Source: three-view drawing plus pictorial views. Frame: mm from the lowest corner of the part. Coordinates: 2 decimals unless noted, no trailing zeros. Write each loop counter-clockwise with the first axis right and the second up, starting at its lowest first coordinate (ties: lowest second). Pieces come first, ordered by that corner, then holes. Notation, with made-up numbers: (81.5, 68.5) -> (120.5, 68.5) arc R19 ccw to (120.5, 83.5) -> close; hole circle Ø10 at (3, -5). An arc over 180 degrees is marked (long way). One line per item, written item: value.
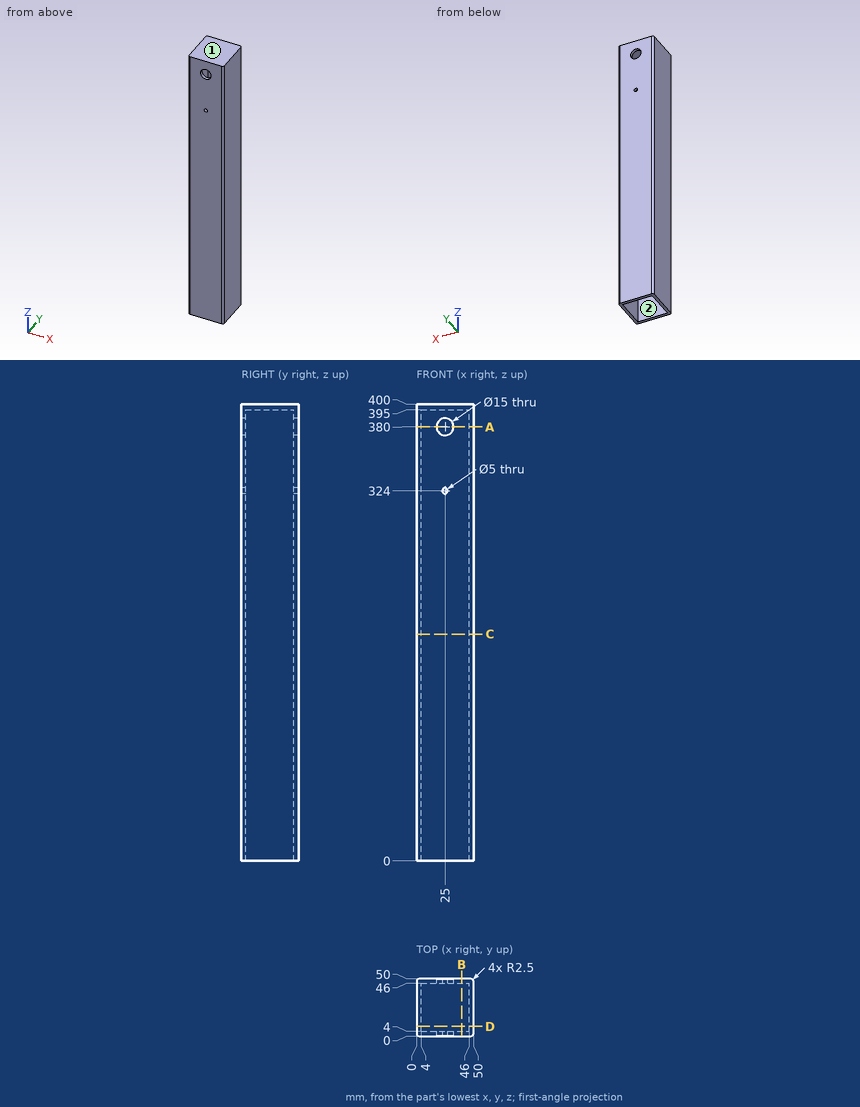
(1) Section C-C (z = 198.5). Return the cut outline in (x, y).
Responses:
outline: (0, 2.5) arc R2.5 ccw to (2.5, 0) -> (47.5, 0) arc R2.5 ccw to (50, 2.5) -> (50, 47.5) arc R2.5 ccw to (47.5, 50) -> (2.5, 50) arc R2.5 ccw to (0, 47.5) -> close; hole (4, 4) -> (46, 4) -> (46, 46) -> (4, 46) -> close
(2) Section B-B (x = 39.5). Return the cut outline in (y, z), then the cut area to 3 significant figures.
Responses:
outline: (0, 0) -> (4, 0) -> (4, 395) -> (46, 395) -> (46, 0) -> (50, 0) -> (50, 400) -> (0, 400) -> close
area: 3,410 mm2
(3) Line query: line 1 (Z direction, x = 25, y = 1.4); line 2 (Y direction, x = 14, z = 237.5). Output: solid intervals per line, ascending. Write a range as [from, to].
Responses:
line 1: z = [0, 321.5], [326.5, 372.5], [387.5, 400]
line 2: y = [0, 4], [46, 50]
(4) Pull-direction query (Z, two-part tool) for the marked faces 1 and 2; classes: released by +Z, released by -Z, zero draft, split by the parting line, or undercut.
Responses:
face 1: released by +Z
face 2: zero draft
(5) Section A-A (z = 380). Return the cut outline in (x, y), then the cut area to 3 significant figures.
Responses:
outline: (0, 2.5) arc R2.5 ccw to (2.5, 0) -> (17.5, 0) -> (17.5, 4) -> (4, 4) -> (4, 46) -> (17.5, 46) -> (17.5, 50) -> (2.5, 50) arc R2.5 ccw to (0, 47.5) -> close; (32.5, 0) -> (47.5, 0) arc R2.5 ccw to (50, 2.5) -> (50, 47.5) arc R2.5 ccw to (47.5, 50) -> (32.5, 50) -> (32.5, 46) -> (46, 46) -> (46, 4) -> (32.5, 4) -> close
area: 611 mm2
